Check sheet for the modelled part. Datum: model origin and axes. Units: mm. A direction names the side the tool comes from. Coordinates: 2 decimals unless noted, no trailing zeros. Loops run counter-clockwise (first coordinate to the right, second up) from the corner with the lowest first, then second, coordinate; pieces in that order, holes last. Notation, with made-up numbers: (55.5, -6) -> (79.5, -6) arc R12 cw to (79.5, 3) -> close; hole circle Ø11 at (79, 17). An arc over 180 degrees is marked (long way). Use CSV: the item, a comma, the result in double quotes. Start each with the question number.
1. Release check for a two-part mould opening along Z. For faces 4 (the face through (-7.509, 157.886, -23.846)), 5 (the face through (-0.3, 20, 57.4)), 6 (the face through (34.168, 164.52, 7.587)) record: pulls with the +Z half, pulls with the -Z half, needs draft (parallel to the pull), parting line crosses it, or undercut.
2. Sectioned sample at B-B, the plane x = 0. Record the cut outline in (y, z), and give its area (3 significant figures).
3. Sectioned sample at D-D, the plane y = 52. Record the cut outline in (x, z), and give its area (3 significant figures).
4. Gauge pin test, flat ends, axial feed: pin 1 (1.5 mm diameter, centred on x = 7.5, y = 131.5, fed in from +Z); pin 2 (5 mm diameter, centred on y = 151.5, z = -12.5, fed in from -X); pin 3 (12 mm diameter, centred on x = 55.5, z = -54.5, fed in from +Y); pin 4 (1 mm diameter, centred on y = 67.5, z = -30.5, fed in from +X). Record the tip position at first contact, or that the pin passes through.
5. Sectioned sample at C-C, the plane y = 164. Record the cut outline in (x, z), and give its area (3 significant figures).
6. Set-up check for faces 1 (the face through (68.335, 10.14, 15.175)), 2 (the face through (-39, 3, -18)), 3 (the face through (34, 145, 0)): record each of +Z, -Z, +X, -X, +Y, -Y from which the full face is reachable in a straight line by a thin tool's end or side.
7. Thickness scan on L1, parallel to X at y = 161, z = 0; L2, parallel to Z at x = -0.5, y = 144 (3 decimals); L3, parallel to Y at x = 29.5, z = -53. Record the ranges inside material, lowest first.
8. Sectioned sample at A-A, the plane z = 0. Record the cut outline in (x, y), and give its area (3 significant figures).
```python
from build123d import *


with BuildPart() as part:
    # Sketch2 → 01_Body (revolve)
    with BuildSketch(Plane.XY, mode=Mode.PRIVATE) as f_01_body_sk:
        with BuildLine():
            Line((70, 0), (70, 20))
            Line((70, 20), (57.013395021, 20))
            ThreePointArc((57.013395021, 20), (51.73965579, 21.984380786), (49.082193259, 26.953081368))
            Line((49.082193259, 26.953081368), (33.5, 145))
            Line((33.5, 145), (35, 145))
            Line((35, 145), (35, 183.5))
            ThreePointArc((35, 183.5), (34.560660172, 184.560660172), (33.5, 185))
            Line((33.5, 185), (26.5, 185))
            ThreePointArc((26.5, 185), (25.439339828, 184.560660172), (25, 183.5))
            Line((25, 183.5), (25, 132.979213819))
            Line((25, 132.979213819), (42.157256224, 3))
            Line((42.157256224, 3), (47, 3))
            ThreePointArc((47, 3), (49.121320344, 2.121320344), (50, 0))
            Line((50, 0), (70, 0))
        make_face()
    revolve(f_01_body_sk.sketch.rotate(Axis((0, 0, 0), (0, 1, 0)), 90), axis=Axis((0, 0, 0), (0, 1, 0)))


solid = part.part
```
Completed:
1,face 4,"undercut"
1,face 5,"needs draft"
1,face 6,"parting line crosses it"
2,outline,"(0, -70) -> (20, -70) -> (20, -57.01) arc R8 cw to (26.95, -49.08) -> (145, -33.5) -> (145, -35) -> (183.5, -35) arc R1.5 ccw to (185, -33.5) -> (185, -26.5) arc R1.5 ccw to (183.5, -25) -> (132.98, -25) -> (3, -42.16) -> (3, -47) arc R3 cw to (0, -50) -> close; (0, 50) arc R3 cw to (3, 47) -> (3, 42.16) -> (132.98, 25) -> (183.5, 25) arc R1.5 ccw to (185, 26.5) -> (185, 33.5) arc R1.5 ccw to (183.5, 35) -> (145, 35) -> (145, 33.5) -> (26.95, 49.08) arc R8 cw to (20, 57.01) -> (20, 70) -> (0, 70) -> close"
2,area,"4,430 mm²"
3,outline,"circle Ø91.55 at (0, 0); hole circle Ø71.38 at (0, 0)"
3,area,"2,580 mm²"
4,pin 1,"z = 34.66"
4,pin 2,"x = -33.54"
4,pin 3,"through"
4,pin 4,"x = 31.83"
5,outline,"circle Ø70 at (0, 0); hole circle Ø50 at (0, 0)"
5,area,"1,880 mm²"
6,face 1,"+Y, -Y"
6,face 2,"-Y"
6,face 3,"none"
7,L1,"-35 to -25, 25 to 35"
7,L2,"-33.628 to -24.995, 24.995 to 33.628"
7,L3,"0 to 20"
8,outline,"(-70, 0) -> (-50, 0) arc R3 cw to (-47, 3) -> (-42.16, 3) -> (-25, 132.98) -> (-25, 183.5) arc R1.5 ccw to (-26.5, 185) -> (-33.5, 185) arc R1.5 ccw to (-35, 183.5) -> (-35, 145) -> (-33.5, 145) -> (-49.08, 26.95) arc R8 cw to (-57.01, 20) -> (-70, 20) -> close; (25, 132.98) -> (42.16, 3) -> (47, 3) arc R3 cw to (50, 0) -> (70, 0) -> (70, 20) -> (57.01, 20) arc R8 cw to (49.08, 26.95) -> (33.5, 145) -> (35, 145) -> (35, 183.5) arc R1.5 ccw to (33.5, 185) -> (26.5, 185) arc R1.5 ccw to (25, 183.5) -> close"
8,area,"4,430 mm²"
